The listing builds one solid part. Answer for the finished solid, in the listing's coordinates (mm). A direction names the side the tool comes from. Give positions to 0.01 mm unless a question says otherwise; leave off trailing zeros. Write each loop counter-clockwise with the first axis right and the second up, starting at its lowest first coordinate (ties: lowest second). Pieces come first, ordered by that corner, then holes.
Autodesk Inventor part; units mm, degrees
ref_plane "YZ Plane" through (0, 0, 0) normal (1, 0, 0) x (0, 1, 0)
ref_plane "XZ Plane" through (0, 0, 0) normal (0, 1, 0) x (-1, 0, 0)
ref_plane "XY Plane" through (0, 0, 0) normal (0, 0, 1) x (1, 0, 0)
sketch "Sketch2" plane through (0, 0, 0) normal (0, 0, 1) x (1, 0, 0)
  line L0 (0, 0) -> (5, 0) construction
  line L1 (40.2, 0) -> (40.2, -40)
  line L2 (40.2, -40) -> (0, -40)
  line L3 (0, -40) -> (0, -13.1)
  arc A0 (31.6412, 0) -> (8.5588, 0) centre (20.1, 8.1) ccw construction
  line L4 (31.6412, 0) -> (40.2, 0)
  line L5 (8.5588, 0) -> (31.6412, 0) construction
  arc A1 (8.5588, 0) -> (31.6412, 0) centre (20.1, 8.1) ccw
  line L6 (35.2, 0) -> (31.6412, 0)
  line L7 (5, 0) -> (5, -13.1)
  line L8 (5, -35) -> (35.2, -35)
  line L9 (35.2, -35) -> (35.2, 0)
  line L10 (0, -13.1) -> (5, -13.1)
  line L11 (0, -13.1) -> (0, 0) construction
  line L12 (5, -13.1) -> (5, -35)
  line L13 (5, 0) -> (8.5588, 0)
  line L14 (8.5588, 0) -> (5, 0)
  line L15 (31.6412, 0) -> (8.5588, 0) construction
  line L16 (20.1, 0) -> (20.1, 8.1)
  line L17 (31.1, -37.2) -> (40.2, -37.2) construction
  line L18 (9.1, -37.2) -> (0, -37.2) construction
  point P0 (2.8, -31.9)
  point P1 (37.4, -9.9)
  dimension "d0" = 40
  dimension "d1" = 40.2
  dimension "d55" = 28.2
  dimension "d56" = 5
  dimension "d57" = 5
  dimension "d58" = 5
  dimension "d59" = 26.9
  dimension "d66" = 48.1
  dimension "d67" = 2.8
  dimension "d68" = 2.8
  dimension "d69" = 2.8
  dimension "d70" = 22
  dimension "d72" = 30.1
  dimension "d73" = 8.1
  dimension "d74" = 2.8
extrude "Extrusion6" add sketch "Sketch2" along normal blind 6.5 contours L1 L2 L3 L10 L12 L8 L9 L4
extrude "Extrusion8" add sketch "Sketch2" along normal blind 2.8 contours L9 L8 L12 L7 L13 A1 L4
hole "Hole2" at (20.1, 8.1, 0) at (31.1, -37.2, 0) at (9.1, -37.2, 0) at (2.8, -31.9, 0) at (37.4, -9.9, 0) direction (0, 0, 1) diameter 2.5 end through all counterbore diameter 4.5 counterbore depth 3
fillet "Fillet1" radius 0.5 9 edges at (40.2, 0, 3.25) (35.2, 0, 4.65) (5, -13.1, 4.65) (5, -13.1, 1.4) (0, -13.1, 3.25) (0, -40, 3.25) (31.6412, 0, 1.4) (8.5588, 0, 1.4) (5, 0, 1.4)
fillet "Fillet2" radius 3 2 edges at (35.2, -35, 4.65) (5, -35, 4.65)
fillet "Fillet3" radius 8 1 edges at (40.2, -40, 3.25)
ref_plane "Work Plane1" through (-4.5, -39.5, 0) normal (-1, 0, 0) x (0, 0, 1)
equation "\"d1\" = side_to_side_outside_dist"
equation "\"d56\" = outside_inside_dist - tol"
equation "\"d57\" = outside_inside_dist - tol"
equation "\"d58\" = outside_inside_dist - tol"
equation "\"d66\" = front_to_axe"
equation "\"d67\" = holes_to_side"
equation "\"d68\" = holes_to_side"
equation "\"d60\" = outside_depth"
equation "\"outside_inside_dist\" = 5.1"
equation "\"outside_depth\" = 6.5"
equation "\"inside_depth\" = outside_depth - inside_to_outside"
equation "\"tol\" = 0.1"
equation "\"side_to_side_outside_dist\" = 40.2"
equation "\"front_to_torsebas\" = 27.1"
equation "\"front_to_axe\" = 48.1"
equation "\"palonnier_diameter\" = 28"
equation "\"holes_to_side\" = 2.8"
equation "\"inside_to_outside\" = 3.5"
equation "\"teflon_sheet_thickness\" = 10.5"
equation "\"stock_top_offset\" = teflon_sheet_thickness - outside_depth"
properties part number "high_leg_teflon_left"
Item 1: Consider probe 1 along X at (y, z) = (-31.9, 5.7); probe 2 along X at (y, z) = (-17, 3.75); probe 3 along X at (y, z) = (-37.2, 2.25). Determine where each line is inside the solid, lowest interval first.
Conclusion:
probe 1: x = 0 to 1.55, 4.05 to 5, 35.2 to 40.2
probe 2: x = 0 to 5, 35.2 to 40.2
probe 3: x = 0 to 6.85, 11.35 to 28.85, 33.35 to 38.28
Item 2: Determine the mould class of faces 1 (the face through (37.794, -37.719, 3.296)), 2 (the face through (5, -6, 1)), 3 (the face through (2, -13.1, 3)), 4 (the face through (31.001, -39.448, 1.521)) for opening direction X: pulls with the +X half, pulls with the -X half, needs draft (parallel to the pull), parting line crosses it, or undercut.
Conclusion:
face 1: pulls with the +X half
face 2: pulls with the -X half
face 3: needs draft
face 4: undercut
Item 3: A cutting plane is placed at D-D, the plane y = -5. Give the vertices of the cut face in (x, z), plus the area to 3 significant figures.
Conclusion:
outline: (5, 0) - (14.88, 0) - (14.88, 2.8) - (5, 2.8) - close; (25.32, 0) - (40.2, 0) - (40.2, 6.5) - (35.2, 6.5) - (35.2, 2.8) - (25.32, 2.8) - close
area: 87.9 mm2
Item 4: A cutting plane is placed at C-C, the plane y = -9.9. Give the vertices of the cut face in (x, z), plus the area to 3 significant figures.
Conclusion:
outline: (5, 0) - (35.15, 0) - (35.15, 2.8) - (5, 2.8) - close; (35.2, 3) - (36.15, 3) - (36.15, 6.5) - (35.2, 6.5) - close; (38.65, 3) - (39.65, 3) - (39.65, 0) - (40.2, 0) - (40.2, 6.5) - (38.65, 6.5) - close
area: 94.8 mm2
Item 5: Each of these flat-tipped pins is pushed along its axis until it touches: P1, Ø2, axis at y = -6, z = 2, coming from the -X side; P2, Ø1.8, axis at x = 19.5, z = 4, coming from the +Y side; P3, Ø3, axis at x = 31.1, y = -37.2, coming from the -Z side. Where does it stop, or does it pass through?
Conclusion:
P1: stops at x = 5
P2: stops at y = -35
P3: stops at z = 3
Item 6: Which of the six approach directions +Z, -Z, +X, -X, +Y, -Y give full straight-line access (tool end or side, diameter ignored) to faces 5 (the face through (10, -36, 3)), 6 (the face through (5.86, -34.1, 4.68)), 7 (the face through (30.046, -36.528, 4.774))?
Conclusion:
face 5: -Z
face 6: +Z, +Y
face 7: +Z, -Z
Item 7: A cutting plane is placed at A-A, the plane x = 2.8. Give the vertices of the cut face in (y, z), plus the area to 3 significant figures.
Conclusion:
outline: (-40, 0) - (-34.15, 0) - (-34.15, 3) - (-33.15, 3) - (-33.15, 6.5) - (-40, 6.5) - close; (-30.65, 3) - (-29.65, 3) - (-29.65, 0) - (-13.1, 0) - (-13.1, 6.5) - (-30.65, 6.5) - close
area: 153 mm2
Item 8: A cutting plane is placed at B-B, the plane z = 0.75. Give the vertices of the cut face in (x, y), plus the area to 3 significant figures.
Conclusion:
outline: (0, -39.5) arc R0.5 ccw to (0.5, -40) - (32.2, -40) arc R8 ccw to (40.2, -32) - (40.2, -0.5) arc R0.5 ccw to (39.7, 0) - (31.9, 0) arc R0.5 ccw to (31.49, -0.21) arc R14.1 cw to (8.71, -0.21) arc R0.5 ccw to (8.3, 0) - (5.5, 0) arc R0.5 ccw to (5, -0.5) - (5, -12.6) arc R0.5 cw to (4.5, -13.1) - (0.5, -13.1) arc R0.5 ccw to (0, -13.6) - close; hole circle Ø4.5 at (2.8, -31.9); hole circle Ø4.5 at (9.1, -37.2); hole circle Ø4.5 at (31.1, -37.2); hole circle Ø4.5 at (37.4, -9.9)
area: 1,370 mm2
